from build123d import *

# Parameters (mm, degrees)
F0_W      = 115
F0_H      = 165.8
F0_R      = 4
F0_R_2    = 2.5
F1_DEPTH  = 5
F2_W      = 18.7665516138
F2_H      = 5
F2_W_2    = 6.2334483862
F3_DEPTH  = 40
F4_W      = 3
F4_H      = 25
F5_DEPTH  = 25
F9_W      = 3
F9_H      = 5
F10_DEPTH = 14.58
F12_DEPTH = 3
F13_W     = 96.2334483862
F13_H     = 9
F14_DEPTH = 5
F15_W     = 96.2334483862
F15_H     = 3
F16_DEPTH = 6
F17_R     = 5
F18_R     = 2


with BuildPart() as f1:
    # F0 (on Top) → F1 (new body)
    with BuildSketch(Plane.XY):
        with Locations((-57.5, 82.9)):
            Rectangle(F0_W, F0_H)
        with Locations((-100, 37.8)):
            Circle(F0_R, mode=Mode.SUBTRACT)
        with Locations((-41.5, 37.8)):
            Circle(F0_R, mode=Mode.SUBTRACT)
        Polygon((-84.125764668, 141.0401467979), (-30, 141.0401467979), (-30, 55), (-58.2305043936, 55), (-58.2305043936, 20), (-84.125764668, 20), align=None, mode=Mode.SUBTRACT)
        with Locations((-100, 93.8)):
            Circle(F0_R_2, mode=Mode.SUBTRACT)
        with Locations((-100, 148.8)):
            Circle(F0_R_2, mode=Mode.SUBTRACT)
        with Locations((-15, 93.8)):
            Circle(F0_R_2, mode=Mode.SUBTRACT)
        with Locations((-15, 148.8)):
            Circle(F0_R_2, mode=Mode.SUBTRACT)
    extrude(amount=-F1_DEPTH)

    # F2 (on face) → F3 (join)
    with BuildSketch(Plane(origin=(0, 0, -5), x_dir=(1, 0, 0), z_dir=(0, 0, -1))):
        with Locations((-105.6167241931, -2.5)):
            Rectangle(F2_W, F2_H)
        with Locations((-118.1167241931, -2.5)):
            Rectangle(F2_W_2, F2_H)
    extrude(amount=F3_DEPTH)

    # F4 (on face) → F5 (join)
    with BuildSketch(Plane(origin=(0, 5, 0), x_dir=(-1, 0, 0), z_dir=(0, 1, 0))):
        with Locations((97.7334483862, -17.5)):
            Rectangle(F4_W, F4_H)
    extrude(amount=F5_DEPTH)


with BuildPart() as f7_1:
    # F7: instance of F1
    add(f1.part.mirror(Plane.XY))

    # F9 (on face) → F10 (join)
    with BuildSketch(Plane.XY.offset(30)):
        with Locations((-97.7334483862, 7.5)):
            Rectangle(F9_W, F9_H)
    extrude(amount=F10_DEPTH)

    # F11 (on face) → F12 (cut, through all)
    with BuildSketch(Plane(origin=(-99.2334483862, 0, 0), x_dir=(0, -1, 0), z_dir=(-1, 0, 0))):
        Polygon((-30, 30), (-30, 5), (-10, 30), align=None)
    extrude(amount=-F12_DEPTH, mode=Mode.SUBTRACT)

    # F13 (on face) → F14 (cut, through all)
    with BuildSketch(Plane.XY.offset(5)):
        with Locations((-48.1167241931, 4.5)):
            Rectangle(F13_W, F13_H)
    extrude(amount=-F14_DEPTH, mode=Mode.SUBTRACT)

    # F15 (on face) → F16 (join)
    with BuildSketch(Plane.XY.offset(5)):
        with Locations((-48.1167241931, 10.5)):
            Rectangle(F15_W, F15_H)
    extrude(amount=F16_DEPTH)

    # F17
    f17_edges = [f7_1.edges().sort_by_distance(p)[0] for p in [
        (-97.733448, 10, 30),
        (-105.616724, 0, 0),
        (-96.233448, 2.5, 45),
        (-121.233448, 2.5, 45),
        (-121.233448, 2.5, 5),
        (-115, 165.8, 2.5),
        (0, 165.8, 2.5),
        (0, 10.5, 11),
        (-58.230504, 55, 2.5),
        (-30, 55, 2.5),
        (-58.230504, 20, 2.5),
        (-84.125765, 20, 2.5),
        (-30, 141.040147, 2.5),
        (-84.125765, 141.040147, 2.5),
        (-48.116724, 9, 0),
    ]]
    fillet(f17_edges, radius=F17_R)

    # F18 (call 1 of 4: OpenCascade refuses the feature's edges together)
    f18_edges = [f7_1.edges().sort_by_distance(p)[0] for p in [
        (-48.116724, 12, 5),
    ]]
    fillet(f18_edges, radius=F18_R)

    # F18#2 (call 2 of 4)
    f18_2_edges = [f7_1.edges().sort_by_distance(p)[0] for p in [
        (-107.116724, 5, 5),
    ]]
    fillet(f18_2_edges, radius=F18_R)

    # F18#3 (call 3 of 4)
    f18_3_edges = [f7_1.edges().sort_by_distance(p)[0] for p in [
        (0, 87.4, 0),
        (-115, 1.464466, 1.464466),
        (-115, 82.9, 0),
        (-113.535534, 164.335534, 0),
        (-57.5, 165.8, 0),
        (-1.464466, 164.335534, 0),
        (-50.616724, 9, 11),
        (0, 9, 5.5),
        (-1.464466, 9, 9.535534),
        (0, 10.464466, 1.464466),
    ]]
    fillet(f18_3_edges, radius=F18_R)

    # F18#4 (call 4 of 4)
    f18_4_edges = [f7_1.edges().sort_by_distance(p)[0] for p in [
        (-30, 98.020073, 0),
        (-57.062882, 141.040147, 0),
        (-82.661299, 139.575681, 0),
        (-31.464466, 139.575681, 0),
        (-84.125765, 80.520073, 0),
        (-82.661299, 21.464466, 0),
        (-31.464466, 56.464466, 0),
        (-71.178135, 20, 0),
        (-44.115252, 55, 0),
        (-59.69497, 21.464466, 0),
        (-56.766038, 53.535534, 0),
        (-58.230504, 37.5, 0),
    ]]
    fillet(f18_4_edges, radius=F18_R)


solid = f7_1.part
Geometry: final body of the model. Coordinates: model frame, mm. A direction names the side the tool comes from. Coordinates: 2 decimals unless noted, no trailing zeros. Loops run counter-clockwise (first coordinate to the right, second up) from the corner with the lowest first, then second, coordinate; pieces in that order, holes last. Notation, with made-up numbers: (43.5, -7.75) - (67.5, -7.75) arc R17 cw to (67.5, 18.25) - close; hole circle Ø2 at (27.5, 20.25). An arc over 180 degrees is marked (long way). One line per question, with ' | ' between items. Start each with the question number.
(1) Reachability of faces 1 (the cylindrical face through (-119.808, 2.465, 6.504)), 2 (the flat face through (-115.4, 1.9, 5)), 3 (the cylindrical face through (-59.66, 21.5, 3.52)), 4 (the flat face through (-109, 0, 25)), 5 (the flat face through (-50, 9, 7)) from +Z, -Z, +X, -X, +Y, -Y: full face, straight path, thin tool, end or side. Return the list, or none.
(2) First-contact query: pin 1 (6 mm diameter, centred on x = -81, y = 68.5, fed in from -Z); pin 2 (3.5 mm diameter, centred on y = 32, z = 4, fed in from -X); pin 3 (4.5 mm diameter, centred on x = -42, z = 9.5, fed in from +Y); pin 4 (1.5 mm diameter, centred on x = -66.5, z = 3.5, fed in from -Y). Flat tips, straight axial feed; report the tip coordinate or a pass-through.
(3) Cut plane A-A on y = 132. Output: boundary loops of the cut face in (x, z).
(4) Cut plane B-B on y = 37.8. Output: boundary loops of the cut face in (x, z), and give its area (3 significant figures).
(5) Cut plane D-D on y = 148.8. Output: boundary loops of the cut face in (x, z), and give its area (3 significant figures).
(6) Draft query along X for faces 6 (the cylindrical face through (-13.85, 146.58, 2.46)), 7 (the flat face through (-49, 12, 9)), 8 (the flat face through (-99.233, 12, 20)), 9 (the flat face through (-96.233, 8, 16)). Return one class per face: +X half, -X half, draft (parallel to the pull), parting line (faces both ways), or undercut.
(7) Cut plane C-C on x = -15. Output: boundary loops of the cut face in (y, z).
(8) Ray query, L1, parallel to X at y = 148.8, z = 1.1; L2, parallel to X at y = 37, z = 1; L3, parallel to Y at x = -104.5, z = 25. Return the intervals inside material, ascending. Write a range as from..to.
Here are the results:
1) face 1: -Z, -X, +Y, -Y | face 2: -Z, -X, -Y | face 3: +Z, -Z | face 4: +Z, -Z, +X, -X, -Y | face 5: +Z, -Z, +X, -Y
2) pin 1: through | pin 2: x = -115 | pin 3: y = 12 | pin 4: y = 9.06
3) outline: (-115, 2) arc R2 ccw to (-113, 0) - (-86.13, 0) arc R2 ccw to (-84.13, 2) - (-84.13, 5) - (-115, 5) - close; (-30, 2) arc R2 ccw to (-28, 0) - (-2, 0) arc R2 ccw to (0, 2) - (0, 5) - (-30, 5) - close
4) outline: (-115, 2) arc R2 ccw to (-113, 0) - (-104, 0) - (-104, 5) - (-115, 5) - close; (-96, 0) - (-86.13, 0) arc R2 ccw to (-84.13, 2) - (-84.13, 5) - (-96, 5) - close; (-58.23, 2) arc R2 ccw to (-56.23, 0) - (-45.5, 0) - (-45.5, 5) - (-58.23, 5) - close; (-37.5, 0) - (-2, 0) arc R2 ccw to (0, 2) - (0, 5) - (-37.5, 5) - close | area: 362 mm²
5) outline: (-115, 2) arc R2 ccw to (-113, 0) - (-102.5, 0) - (-102.5, 5) - (-115, 5) - close; (-97.5, 0) - (-17.5, 0) - (-17.5, 5) - (-97.5, 5) - close; (-12.5, 0) - (-2, 0) arc R2 ccw to (0, 2) - (0, 5) - (-12.5, 5) - close | area: 523 mm²
6) face 6: undercut | face 7: draft | face 8: -X half | face 9: +X half
7) outline: (9, 5) arc R5 ccw to (14, 0) - (91.3, 0) - (91.3, 5) - (14, 5) arc R2 cw to (12, 7) - (12, 11) - (11, 11) arc R2 ccw to (9, 9) - close; (96.3, 0) - (146.3, 0) - (146.3, 5) - (96.3, 5) - close; (151.3, 0) - (163.8, 0) arc R2 ccw to (165.8, 2) - (165.8, 5) - (151.3, 5) - close
8) L1: -114.79..-102.5, -97.5..-17.5, -12.5..-0.21 | L2: -114.73..-103.92, -96.08..-84.39, -57.96..-45.42, -37.58..-0.27 | L3: 0..5
